Model file for the job. Use its own axes, mm. A direction names the side the tool comes from. Give positions to 0.01 mm unless a question says otherwise; leave off trailing zeros. Write each loop counter-clockwise with the first axis right and the second up, starting at its lowest first coordinate (ties: lowest second). Pieces come first, ordered by that corner, then holes. Notation, with made-up numbers: (28.25, -28.5) - (58.25, -28.5) arc R27 ccw to (58.25, 7.5) - close; hole circle Ø11 at (34.25, 45). An arc over 180 degrees is marked (long way). One line per item, written item: value. Start each with the question number.
(1) Cut at B-B, the plane x = 10.5. List the corners of the cut face in (y, z), and give its area (3 significant figures).
(2) Drop flat-ended pins along their axis: P1, Ø10, axis at x = 15, y = 9.5, coming from the +Z side; P2, Ø3, axis at y = -8, z = 11.5, coming from the -X side; P3, Ø12, axis at x = 14.5, z = -9, coming from the +Y side. Give the stop position or say it passes through.
(3) Probe L1, parallel to Z at x = 2.9, y = -6.25; L2, parallel to Y at x = 12, z = 0; L3, parallel to X at y = -2, z = 12. List the from-to ranges inside material, lowest first.
(4) Cut at A-A, the plane y = -15.5. List the corners of the cut face in (x, z).
(5) Mould opens along Y. For faces 1 (the face through (15, -8, 0)), 2 (the face through (15, 11, 0)), 3 (the face through (3.7, 0.36, 32.5)) say: pulls with the +Y half, pulls with the -Y half, needs draft (parallel to the pull), parting line crosses it, or undercut.
(6) Cut at C-C, the plane z = 28. List the corners of the cut face in (x, y), and give its area (3 significant figures).
(7) Cut at D-D, the plane x = 16. List the corners of the cut face in (y, z), and give its area (3 significant figures).
(8) 3-axis set-ups, long thin cutter, end or side, ignore diameter. For faces 4 (the face through (0, -2.4, -2.4)), 5 (the face through (1.6, 0, 29)), 6 (the face through (3.93, -6.11, 7.58)), 7 (the face through (1.6, 0, -29)): which of +Z, -Z, +X, -X, +Y, -Y reach the whole face in a straight line?
from build123d import *

# Parameters (mm, degrees)
CORTAR_EXTRUIR2_DEPTH  = 7.5
CROQUIS5_R             = 1.5
CORTAR_EXTRUIR4_DEPTH  = 25
CORTAR_EXTRUIR14_DEPTH = 1.6
CORTAR_EXTRUIR15_DEPTH = 18
CORTAR_EXTRUIR18_DEPTH = 17.5
CROQUIS21_R            = 1
CORTAR_EXTRUIR19_DEPTH = 12.5
CROQUIS22_R            = 3.25
CORTAR_EXTRUIR20_DEPTH = 5.5


with BuildPart() as part:
    # Croquis1 → Revolución1 (revolve)
    with BuildSketch(Plane(origin=(0, 0, 0), x_dir=(1, 0, 0), z_dir=(0, 1, 0)), mode=Mode.PRIVATE) as revoluci_n1_sk:
        Polygon((0, 0), (25, 0), (25, 20), (7.5, 19.966144384), (7.5, 32.5), (0, 32.5), (0, 20), (2.75, 20), (2.75, 10), (0, 10), align=None)
    revolve(revoluci_n1_sk.sketch.rotate(Axis((0, 0, 0), (1, 0, 0)), 180), axis=Axis((0, 0, 0), (1, 0, 0)))

    # Croquis2 → Cortar-Extruir2 (cut)
    with BuildSketch(Plane.ZY):
        with BuildLine():
            ThreePointArc((-14.142135624, 14.142135624), (0, 20), (14.142135624, 14.142135624))
            Line((14.142135624, 14.142135624), (22.980970389, 22.980970389))
            ThreePointArc((22.980970389, 22.980970389), (0, 32.5), (-22.980970389, 22.980970389))
            Line((-22.980970389, 22.980970389), (-14.142135624, 14.142135624))
        make_face()
        with BuildLine():
            Line((22.980970389, -22.980970389), (14.142135624, -14.142135624))
            ThreePointArc((14.142135624, -14.142135624), (0, -20), (-14.142135624, -14.142135624))
            Line((-14.142135624, -14.142135624), (-22.980970389, -22.980970389))
            ThreePointArc((-22.980970389, -22.980970389), (0, -32.5), (22.980970389, -22.980970389))
        make_face()
    extrude(amount=-CORTAR_EXTRUIR2_DEPTH, mode=Mode.SUBTRACT)

    # Croquis5 → Cortar-Extruir4 (cut)
    with BuildSketch(Plane(origin=(25, 0, 0), x_dir=(0, 0, -1), z_dir=(1, 0, 0))):
        with Locations((0, 12.5)):
            Circle(CROQUIS5_R)
        with Locations((10.825317547, -6.25)):
            Circle(CROQUIS5_R)
        with Locations((-10.825317547, -6.25)):
            Circle(CROQUIS5_R)
    extrude(amount=-CORTAR_EXTRUIR4_DEPTH, mode=Mode.SUBTRACT)

    # Croquis17 → Cortar-Extruir14 (cut)
    with BuildSketch(Plane.ZY):
        with BuildLine():
            Line((26, 0), (32.5, 0))
            ThreePointArc((32.5, 0), (32.469067201, 1.417630089), (32.376327688, 2.832561639))
            Line((32.376327688, 2.832561639), (25.90106215, 2.266049311))
            ThreePointArc((25.90106215, 2.266049311), (25.975253761, 1.134104071), (26, 0))
        make_face()
        with BuildLine():
            ThreePointArc((32.376327688, -2.832561639), (32.469067201, -1.417630089), (32.5, 0))
            Line((32.5, 0), (26, 0))
            ThreePointArc((26, 0), (25.975253761, -1.134104071), (25.90106215, -2.266049311))
            Line((25.90106215, -2.266049311), (32.376327688, -2.832561639))
        make_face()
        with BuildLine():
            Line((-25.90106215, 2.266049311), (-32.376327688, 2.832561639))
            ThreePointArc((-32.376327688, 2.832561639), (-32.469067201, 1.417630089), (-32.5, 0))
            Line((-32.5, 0), (-26, 0))
            ThreePointArc((-26, 0), (-25.975253761, 1.134104071), (-25.90106215, 2.266049311))
        make_face()
        with BuildLine():
            ThreePointArc((-32.5, 0), (-32.469067201, -1.417630089), (-32.376327688, -2.832561639))
            Line((-32.376327688, -2.832561639), (-25.90106215, -2.266049311))
            ThreePointArc((-25.90106215, -2.266049311), (-25.975253761, -1.134104071), (-26, 0))
            Line((-26, 0), (-32.5, 0))
        make_face()
    extrude(amount=-CORTAR_EXTRUIR14_DEPTH, mode=Mode.SUBTRACT)

    # Croquis18 → Cortar-Extruir15 (cut)
    with BuildSketch(Plane.ZY):
        with BuildLine():
            Line((0, 0), (-1.86, 2.48))
            ThreePointArc((-1.86, 2.48), (-1.386362146, -2.772724292), (3.1, 0))
            ThreePointArc((3.1, 0), (2.772724292, 1.386362146), (1.86, 2.48))
            Line((1.86, 2.48), (0, 0))
        make_face()
        Polygon((0, 0), (-1.86, 2.48), (1.86, 2.48), align=None)
    extrude(amount=-CORTAR_EXTRUIR15_DEPTH, mode=Mode.SUBTRACT)

    # Croquis20 → Cortar-Extruir18 (cut)
    with BuildSketch(Plane(origin=(25, 0, 0), x_dir=(0, 0, -1), z_dir=(1, 0, 0))):
        with BuildLine():
            Line((0, -12.5), (-15.612494996, -12.5))
            ThreePointArc((-15.612494996, -12.5), (0, -20), (15.612494996, -12.5))
            Line((15.612494996, -12.5), (0, -12.5))
        make_face()
    extrude(amount=-CORTAR_EXTRUIR18_DEPTH, mode=Mode.SUBTRACT)

    # Croquis21 → Cortar-Extruir19 (cut)
    with BuildSketch(Plane.XZ.offset(12.5)):
        with Locations(Location((16, 0, 0), (0, 0, 270))):
            Circle(CROQUIS21_R)
    extrude(amount=-CORTAR_EXTRUIR19_DEPTH, mode=Mode.SUBTRACT)

    # Croquis22 → Cortar-Extruir20 (cut)
    with BuildSketch(Plane.ZY):
        with Locations((0, 12.5)):
            Circle(CROQUIS22_R)
        with Locations((10.825317547, -6.25)):
            Circle(CROQUIS22_R)
        with Locations((-10.825317547, -6.25)):
            Circle(CROQUIS22_R)
    extrude(amount=-CORTAR_EXTRUIR20_DEPTH, mode=Mode.SUBTRACT)


solid = part.part
Answers follow:
1. outline: (-12.5, -15.58) arc R19.97 ccw (long way) to (-12.5, 15.58) - close; hole circle Ø3 at (-6.25, -10.83); hole circle Ø3 at (-6.25, 10.83); hole (2.48, -1.86) - (2.48, 1.86) arc R3.1 ccw (long way) to start; hole circle Ø3 at (12.5, 0)
1. area: 1,040 mm²
2. P1: stops at z = 19.47
2. P2: stops at x = 2.75
2. P3: stops at y = 19.75
3. L1: z = -31.89 to -14.08, -7.58 to 7.58, 14.08 to 31.89
3. L2: y = -12.5 to -3.1, 2.48 to 11, 14 to 19.97
3. L3: x = 2.75 to 25
4. outline: (0, -28.57) - (7.5, -28.57) - (7.5, -15.5) - (0, -15.5) - close; (0, 15.5) - (7.5, 15.5) - (7.5, 28.57) - (0, 28.57) - close; (2.75, -12.64) - (7.5, -12.64) - (7.5, 12.64) - (2.75, 12.64) - close
5. face 1: needs draft
5. face 2: undercut
5. face 3: parting line crosses it
6. outline: (0, -16.5) - (7.5, -16.5) - (7.5, 16.5) - (0, 16.5) - (0, 2.45) - (1.6, 2.45) - (1.6, -2.45) - (0, -2.45) - close
6. area: 240 mm²
7. outline: (-12.5, -15.59) arc R19.98 ccw (long way) to (-12.5, 15.59) - (-12.5, 1) - (-2.93, 1) arc R3.1 cw to (2.48, 1.86) - (2.48, -1.86) arc R3.1 cw to (-2.93, -1) - (-12.5, -1) - close; hole circle Ø3 at (-6.25, -10.83); hole circle Ø3 at (-6.25, 10.83); hole circle Ø3 at (12.5, 0)
7. area: 1,020 mm²
8. face 4: +Z, -Z, -X, +Y, -Y
8. face 5: +Z, -X
8. face 6: -X
8. face 7: -Z, -X
